from build123d import *

# Parameters (mm, degrees)
SKETCH1_W           = 60
SKETCH1_H           = 53
BOSS_EXTRUDE1_DEPTH = 0.8
CUT_EXTRUDE2_DEPTH  = 0.8
SKETCH3_W           = 10.9
SKETCH3_H           = 21.35
SKETCH3_W_2         = 46.8
SKETCH3_H_2         = 21.5
BOSS_EXTRUDE2_DEPTH = 1
SKETCH4_W           = 10.9
SKETCH4_H           = 5
CUT_EXTRUDE3_DEPTH  = 10


with BuildPart() as part:
    # Sketch1 → Boss-Extrude1 (new body)
    with BuildSketch(Plane.XY):
        with Locations((30, 26.5)):
            Rectangle(SKETCH1_W, SKETCH1_H)
    extrude(amount=BOSS_EXTRUDE1_DEPTH)

    # Sketch2 → Cut-Extrude2 (cut)
    with BuildSketch(Plane.XY.offset(0.8)):
        with BuildLine():
            ThreePointArc((0, 43), (2.928932188, 50.071067812), (10, 53))
            Line((10, 53), (0, 53))
            Line((0, 53), (0, 43))
        make_face()
        with BuildLine():
            ThreePointArc((10, 21.4), (2.928932188, 24.328932188), (0, 31.4))
            Line((0, 31.4), (0, 0))
            Line((0, 0), (21, 0))
            Line((21, 0), (21, 11.4))
            ThreePointArc((21, 11.4), (18.071067812, 18.471067812), (11, 21.4))
            Line((11, 21.4), (10, 21.4))
        make_face()
        with BuildLine():
            Line((60, 0), (60, 31.4))
            ThreePointArc((60, 31.4), (57.071067812, 24.328932188), (50, 21.4))
            Line((50, 21.4), (49, 21.4))
            ThreePointArc((49, 21.4), (41.928932188, 18.471067812), (39, 11.4))
            Line((39, 11.4), (39, 0))
            Line((39, 0), (60, 0))
        make_face()
        with BuildLine():
            Line((60, 53), (50, 53))
            ThreePointArc((50, 53), (57.071067812, 50.071067812), (60, 43))
            Line((60, 43), (60, 53))
        make_face()
    extrude(amount=-CUT_EXTRUDE2_DEPTH, mode=Mode.SUBTRACT)

    # Sketch3 → Boss-Extrude2 (add)
    with BuildSketch(Plane.XY.offset(0.8)):
        with Locations((30, 15.775)):
            Rectangle(SKETCH3_W, SKETCH3_H)
        with Locations((30, 37.2)):
            Rectangle(SKETCH3_W_2, SKETCH3_H_2)
    extrude(amount=BOSS_EXTRUDE2_DEPTH)

    # Sketch4 → Cut-Extrude3 (cut)
    with BuildSketch(Plane.XY.offset(1.8)):
        with Locations((30, 7.6)):
            Rectangle(SKETCH4_W, SKETCH4_H)
    extrude(amount=-CUT_EXTRUDE3_DEPTH, mode=Mode.SUBTRACT)


solid = part.part
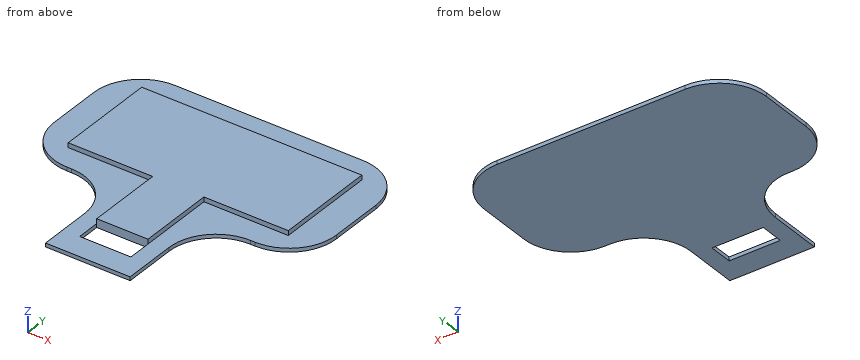
Could you check a few things on this model? Use its own coordinates, in mm. Give positions to 0.01 mm unless a question says otherwise; leave off trailing zeros. Loops run counter-clockwise (first coordinate to the right, second up) from the corner with the lowest first, then second, coordinate; pieces in that order, holes last. Notation, with made-up numbers: M 67,63.25 L 83,63.25 A21 cw 83,71.25 Z; hole C -27.5,41.5 d9. An arc over 180 degrees is marked long. Answer as a JSON object with one key per item and string values.
Q1. Suppose I cut it at C-C, the plane z = 1.1. List the corners of the cut face in (x, y) for me.
Values found:
{"outline": "M 6.6,26.45 L 24.55,26.45 L 24.55,10.1 L 35.45,10.1 L 35.45,26.45 L 53.4,26.45 L 53.4,47.95 L 6.6,47.95 Z"}
Q2. Suppose I cut it at D-D, the plane y = 25. List the corners of the cut face in (x, z) for me.
Values found:
{"outline": "M 2.32,0 L 57.68,0 L 57.68,0.8 L 35.45,0.8 L 35.45,1.8 L 24.55,1.8 L 24.55,0.8 L 2.32,0.8 Z"}
Q3. For P1, Ø0.6, axis at x = 49.5, z = 0.5, coming from the -Y side; P2, Ø0.9, axis at y = 3.5, z = 0.5, coming from the -X side; P3, Ø0.5, axis at x = 21.5, z = 1.5, coming from the +Y side, each with a flat end and sliding along its axis, tell me the tip position at first contact or that it passes through.
Values found:
{"P1": "stops at y = 21.4", "P2": "stops at x = 21", "P3": "stops at y = 47.95"}
Q4. Suppose I cut it at A-A, the plane x = 34. List the corners of the cut face in (y, z) for me.
Values found:
{"outline": "M 0,0 L 5.1,0 L 5.1,0.8 L 0,0.8 Z; M 10.1,0 L 53,0 L 53,0.8 L 47.95,0.8 L 47.95,1.8 L 10.1,1.8 Z"}
Q5. If I drill on probe 1 along Y at (x, z) = (29, 0.35); probe 2 along Y at (x, z) = (31, 1.35); probe 3 along X at (y, z) = (44.5, 0.85), over which ranges is the centre line in solid material (lowest first)? Write a range as [from, to].
Values found:
{"probe 1": "y = [0, 5.1], [10.1, 53]", "probe 2": "y = [10.1, 47.95]", "probe 3": "x = [6.6, 53.4]"}
Q6. Suppose I cut it at B-B, the plane y = 9. List the corners of the cut face in (x, z) for me.
Values found:
{"outline": "M 21,0 L 24.55,0 L 24.55,0.8 L 21,0.8 Z; M 35.45,0 L 39,0 L 39,0.8 L 35.45,0.8 Z"}
